from build123d import *

# Parameters (mm, degrees)
MODEL_R                 = 1.5
SALIENTE_EXTRUIR1_DEPTH = 3


with BuildPart() as part:
    # Model → Saliente-Extruir1 (new body)
    with BuildSketch(Plane.XY):
        with BuildLine():
            Line((-105.943383637, 101.056539338), (-105.943383637, 65.056539338))
            ThreePointArc((-105.943383637, 65.056539338), (-104.625364152, 61.874558823), (-101.443383637, 60.556539338))
            Line((-101.443383637, 60.556539338), (-65.443383637, 60.556539338))
            ThreePointArc((-65.443383637, 60.556539338), (-63.721308191, 60.899081442), (-62.261403122, 61.874558823))
            Line((-62.261403122, 61.874558823), (-104.625364152, 104.238519853))
            ThreePointArc((-104.625364152, 104.238519853), (-105.600841533, 102.778614784), (-105.943383637, 101.056539338))
        make_face()
        with Locations((-101.443383637, 92.056539338)):
            Circle(MODEL_R, mode=Mode.SUBTRACT)
        with Locations((-101.443383637, 83.056539338)):
            Circle(MODEL_R, mode=Mode.SUBTRACT)
        with Locations((-92.443383637, 83.056539338)):
            Circle(MODEL_R, mode=Mode.SUBTRACT)
        with Locations((-101.443383637, 74.056539338)):
            Circle(MODEL_R, mode=Mode.SUBTRACT)
        with Locations((-92.443383637, 74.056539338)):
            Circle(MODEL_R, mode=Mode.SUBTRACT)
        with Locations((-83.443383637, 74.056539338)):
            Circle(MODEL_R, mode=Mode.SUBTRACT)
        with Locations((-101.443383637, 65.056539338)):
            Circle(MODEL_R, mode=Mode.SUBTRACT)
        with Locations((-92.443383637, 65.056539338)):
            Circle(MODEL_R, mode=Mode.SUBTRACT)
        with Locations((-83.443383637, 65.056539338)):
            Circle(MODEL_R, mode=Mode.SUBTRACT)
        with Locations((-74.443383637, 65.056539338)):
            Circle(MODEL_R, mode=Mode.SUBTRACT)
    extrude(amount=SALIENTE_EXTRUIR1_DEPTH)


solid = part.part
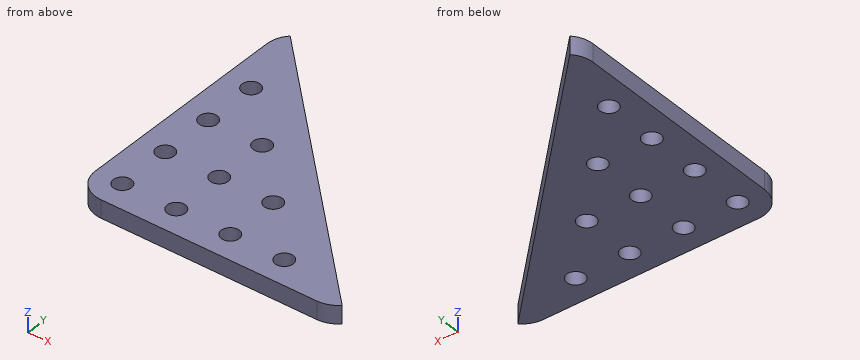
Here's how the part is built. I have some questions about the finished solid (model axes, mm). Give positions to 0.01 mm unless a question says otherwise; leave off trailing zeros. Loops run counter-clockwise (first coordinate to the right, second up) from the corner with the lowest first, then second, coordinate; pieces in that order, holes last. Notation, with made-up numbers: (71, 34.25) -> (116, 34.25) arc R17 cw to (116, 49.25) -> close; hole circle Ø9 at (-7, 34). An arc over 180 degrees is marked (long way). One line per item, written item: value.
Q1. Suppose I cut it at B-B on x = -92. Please give me the cut outline in (y, z), then the cut area to 3 significant figures.
Answers follow:
outline: (60.56, 0) -> (63.62, 0) -> (63.62, 3) -> (60.56, 3) -> close; (66.49, 0) -> (72.62, 0) -> (72.62, 3) -> (66.49, 3) -> close; (75.49, 0) -> (81.62, 0) -> (81.62, 3) -> (75.49, 3) -> close; (84.49, 0) -> (91.61, 0) -> (91.61, 3) -> (84.49, 3) -> close
area: 67.4 mm^2
Q2. Suppose I cut it at A-A on y = 75. Please give me the cut outline in (x, z).
Answers follow:
outline: (-105.94, 0) -> (-102.61, 0) -> (-102.61, 3) -> (-105.94, 3) -> close; (-100.28, 0) -> (-93.61, 0) -> (-93.61, 3) -> (-100.28, 3) -> close; (-91.28, 0) -> (-84.61, 0) -> (-84.61, 3) -> (-91.28, 3) -> close; (-82.28, 0) -> (-75.39, 0) -> (-75.39, 3) -> (-82.28, 3) -> close
Q3. Suppose I cut it at C-C on x = -102. Please give me the cut outline in (y, z).
Answers follow:
outline: (60.59, 0) -> (63.66, 0) -> (63.66, 3) -> (60.59, 3) -> close; (66.45, 0) -> (72.66, 0) -> (72.66, 3) -> (66.45, 3) -> close; (75.45, 0) -> (81.66, 0) -> (81.66, 3) -> (75.45, 3) -> close; (84.45, 0) -> (90.66, 0) -> (90.66, 3) -> (84.45, 3) -> close; (93.45, 0) -> (101.61, 0) -> (101.61, 3) -> (93.45, 3) -> close
Q4. If I drill on line 1 along Y through (x, z) = (-92.5, 2.25); line 2 along X through (y, z) = (73.5, 1.8); line 3 along Y through (x, z) = (-92, 2.6), over which ranges is the centre line in solid material (lowest first)?
Answers follow:
line 1: 60.56 to 63.56, 66.56 to 72.56, 75.56 to 81.56, 84.56 to 92.11
line 2: -105.94 to -102.84, -100.05 to -93.84, -91.05 to -84.84, -82.05 to -73.89
line 3: 60.56 to 63.62, 66.49 to 72.62, 75.49 to 81.62, 84.49 to 91.61
Q5. Suppose I cut it at D-D on z = 2.15. State how many separate pieces and enclosed holes the cut face has, then the cut area to 3 significant figures.
Answers follow:
separate pieces: 1
enclosed holes: 10
area: 933 mm^2
